Autodesk Inventor part; units mm, degrees
ref_plane "YZ Plane" through (0, 0, 0) normal (1, 0, 0) x (0, 1, 0)
ref_plane "XZ Plane" through (0, 0, 0) normal (0, 1, 0) x (-1, 0, 0)
ref_plane "XY Plane" through (0, 0, 0) normal (0, 0, 1) x (1, 0, 0)
sketch "Skizze1" plane through (0, 0, 0) normal (0, 0, 1) x (1, 0, 0)
  line L0 (-27.5, -31.25) -> (27.5, -31.25)
  line L1 (27.5, -31.25) -> (27.5, 31.25)
  line L2 (27.5, 31.25) -> (-27.5, 31.25)
  line L3 (-27.5, 31.25) -> (-27.5, -31.25)
  point P0 (0, 0)
  point P1 (-27.5, 0)
  point P2 (0, -31.25)
  dimension "d5" = 55
  dimension "d6" = 62.5
extrude "Extrusion1" add sketch "Skizze1" along normal blind 30
sketch "Skizze2" plane through (0, 0, 30) normal (0, 0, 1) x (1, 0, 0)
  line L0 (-22.5, -26.25) -> (22.5, -26.25)
  line L1 (22.5, -26.25) -> (22.5, 26.25)
  line L2 (22.5, 26.25) -> (-22.5, 26.25)
  line L3 (-22.5, 26.25) -> (-22.5, -26.25)
  point P0 (0, 0)
  point P1 (0, 26.25)
  point P2 (-22.5, 0)
  dimension "d3" = 45
  dimension "d4" = 52.5
hole "Bohrung1" at (-22.5, 26.25, 30) at (-22.5, -26.25, 30) at (22.5, -26.25, 30) at (22.5, 26.25, 30) direction (0, 0, -1) diameter 6 end through all
sketch "Skizze3" plane through (0, 0, 30) normal (0, 0, 1) x (1, 0, 0)
  circle A0 centre (0, 0) radius 27.5
  circle A1 centre (22.5, -26.25) radius 3
  circle A2 centre (-22.5, 26.25) radius 3
  circle A3 centre (-22.5, -26.25) radius 3
  circle A4 centre (22.5, 26.25) radius 3
  line L0 (-27.5, -31.25) -> (27.5, -31.25)
  line L1 (27.5, -31.25) -> (27.5, 31.25)
  line L2 (27.5, 31.25) -> (-27.5, 31.25)
  line L3 (-27.5, 31.25) -> (-27.5, -31.25)
  dimension "d14" = 55
extrude "Extrusion2" cut sketch "Skizze3" against normal blind 25 contours L1 L0 L3 A0 | A0 L3 L2 L1
sketch "Skizze4" plane through (0, 0, 30) normal (0, 0, 1) x (1, 0, 0)
  circle A0 centre (0, 0) radius 23.5
  dimension "d17" = 47
extrude "Extrusion3" cut sketch "Skizze4" against normal through all
fillet "Rundung1" radius 5 4 edges at (-27.5, -31.25, 2.5) (27.5, -31.25, 2.5) (27.5, 31.25, 2.5) (-27.5, 31.25, 2.5)
properties part number "Rohrhalterung"
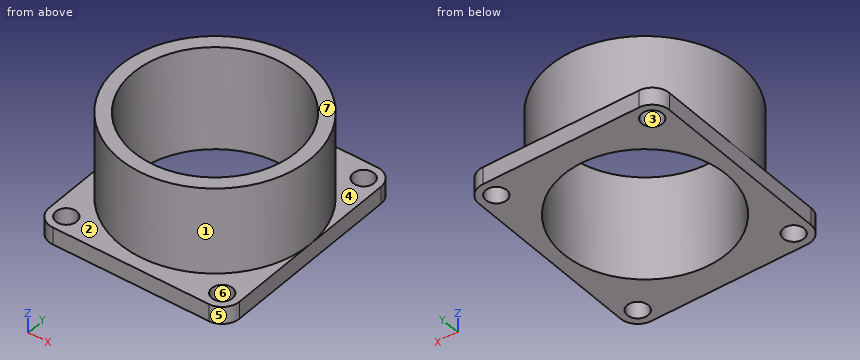
Source: CAD feature listing. Evaluate the final solid. Frame: model axes, mm. Face numbers are marked on the shaded views. A direction names the side the tool comes from. Coordinates: 2 decimals unless noted, no trailing zeros. Order: outer loops, then holes, each group sorted by start corner. A loop starts at its lowest first (then second) coordinate and runs counter-clockwise, first axis right, second up. Notation, with made-up numbers: M 88,-7 L 121,-7 A25 ccw 121,23 Z; hole C 63.5,-1 d6. An arc over 180 degrees is marked long. Write each question's results on one line, items separated by ' | '. Start each with the question number.
1. Section C-C, the plane z = 12.5. Return the cut outline in (x, y).
2. Material intervals for L1, parallel to X at y = 26.25, z = 3.4; L2, parallel to Y at x = 0, z = 24; L3, parallel to X at y = -11, z = 28.5, sorted ascending.
3. Section B-B, the plane y = -9.5. Return the cut outline in (x, z).
4. Draft query along Y for the marked faces 5, 6 and 7. Return one class per face: +Y half, -Y half, draft (parallel to the pull), parting line (faces both ways), or undercut.
5. Reachability of the marked faces 1, 2, 3 and 4 from +Z, -Z, +X, -X, +Y, -Y: full face, straight path, thin tool, end or side. Return the list, or none.
6. Section A-A, the plane x = -4.5. Return the cut outline in (y, z), then the cut area to 3 significant figures.
7. Pin query (flat end, axial travel): pin 1 (5.5 mm diameter, centred on x = -22.5, y = 26.25, fed in from -Z); pin 2 (3 mm diameter, centred on y = -8.5, z = 19.5, fed in from +X); pin 3 (3 mm diameter, centred on y = 21.5, z = 15, fed in from -X); pin 4 (5 mm diameter, centred on y = 11.5, z = 16.5, fed in from -X). Return the tip coordinate at first contact, or that it passes through.
Solution:
1) outline: C 0,0 d55; hole C 0,0 d47
2) L1: -27.5 to -25.5, -19.5 to 19.5, 25.5 to 27.5 | L2: -27.5 to -23.5, 23.5 to 27.5 | L3: -25.2 to -20.77, 20.77 to 25.2
3) outline: M -27.5,0 L -21.49,0 L -21.49,30 L -25.81,30 L -25.81,5 L -27.5,5 Z; M 21.49,0 L 27.5,0 L 27.5,5 L 25.81,5 L 25.81,30 L 21.49,30 Z
4) face 5: -Y half | face 6: undercut | face 7: draft
5) face 1: +Z | face 2: +Z, -Y | face 3: +Z, -Z | face 4: +Z, +Y
6) outline: M -31.25,0 L -23.07,0 L -23.07,30 L -27.13,30 L -27.13,5 L -31.25,5 Z; M 23.07,0 L 31.25,0 L 31.25,5 L 27.13,5 L 27.13,30 L 23.07,30 Z | area: 285 mm²
7) pin 1: through | pin 2: x = 26.59 | pin 3: x = -18.87 | pin 4: x = -25.99
